Check sheet for the modelled part. Datum: model origin and axes. Units: mm. A direction names the side the tool comes from. Round coordinates to 2 decimals unless told otherwise and drop trailing zeros. Order: outer loops, then holes, each group sorted by start corner. A loop starts at its lowest first (then second) coordinate and runs counter-clockwise, first axis right, second up. Notation, with made-up numbers: M -11,-33.5 L 40,-33.5 A23 cw 40,-15.5 Z; hole C 60.25,19 d5. An arc over 180 degrees is marked long. One line per item, written item: value. Start each with the question number.
(1) Thickness scan on L1, parallel to Z at x = -73, y = 71; L2, parallel to X at y = 14, z = 7.75; L3, parallel to X at y = -11, z = 2.5. Record the ranges inside material, lowest first.
(2) Release check for a two-part mould opening along Z. For faces 3 (the face through (-80, 32, 8)), 4 (the face through (-78, -8.4, 12)) record: released by +Z, released by -Z, zero draft, split by the parting line, or undercut.
(3) Access from +Z, -Z, +X, -X, +Y, -Y to the whole of each face (thin tool, end or side, straight path). Record for faces 1 (the face through (-76.666, -33.778, -1.465)), 2 (the face through (-78, 53, 14)).
(4) Cross-section at A-A, the plane y = -32.5. Enter the section's corners in (x, z).
(5) Depth check by flat-ended pin: pin 1 Ø1.2 at (y, z) = (52, 2.5) entering from -X; pin 2 Ø2.5 at (x, y) = (-75, 52.5) entering from +Z. Enter the tip coordinate at first touch or a pass-through.
from build123d import *

# Parameters (mm, degrees)
SKETCH1_W           = 10
SKETCH1_H           = 85
BOSS_EXTRUDE2_DEPTH = 5
SKETCH2_W           = 10
SKETCH2_H           = 170
CUT_EXTRUDE1_DEPTH  = 1
SKETCH3_W           = 5
SKETCH3_H           = 8.2
CUT_EXTRUDE2_DEPTH  = 4
BOSS_EXTRUDE3_DEPTH = 9
SKETCH6_W           = 5
SKETCH6_H           = 170
BOSS_EXTRUDE4_DEPTH = 10
SKETCH7_W           = 10
SKETCH7_H           = 170
BOSS_EXTRUDE6_DEPTH = 5
SKETCH9_W           = 10
SKETCH9_H           = 170
BOSS_EXTRUDE7_DEPTH = 5
SKETCH10_R          = 2.1
CUT_EXTRUDE3_DEPTH  = 39
CUT_EXTRUDE6_DEPTH  = 39
SKETCH14_W          = 10
SKETCH14_H          = 2
CUT_EXTRUDE7_DEPTH  = 39


with BuildPart() as part:
    # Sketch1 → Boss-Extrude2 (new body)
    with BuildSketch(Plane.XY):
        with Locations((-75, 0)):
            Rectangle(SKETCH1_W, SKETCH1_H)
        Polygon((-78.6, 10.4), (-75, 8.4), (-71.4, 10.4), (-71.4, 14.6), (-75, 16.6), (-78.6, 14.6), align=None, mode=Mode.SUBTRACT)
        Polygon((-78.6, 34.6), (-78.6, 30.4), (-75, 28.4), (-71.4, 30.4), (-71.4, 34.6), (-75, 36.6), align=None, mode=Mode.SUBTRACT)
        Polygon((-78.6, -10.4), (-78.6, -14.6), (-75, -16.6), (-71.4, -14.6), (-71.4, -10.4), (-75, -8.4), align=None, mode=Mode.SUBTRACT)
        Polygon((-78.6, -34.6), (-75, -36.6), (-71.4, -34.6), (-71.4, -30.4), (-75, -28.4), (-78.6, -30.4), align=None, mode=Mode.SUBTRACT)
        with Locations((-75, 85)):
            Rectangle(SKETCH1_W, SKETCH1_H)
        Polygon((-78.6, 115.4), (-75, 113.4), (-71.4, 115.4), (-71.4, 119.6), (-75, 121.6), (-78.6, 119.6), align=None, mode=Mode.SUBTRACT)
        Polygon((-78.6, 95.4), (-75, 93.4), (-71.4, 95.4), (-71.4, 99.6), (-75, 101.6), (-78.6, 99.6), align=None, mode=Mode.SUBTRACT)
        Polygon((-78.6, 50.4), (-75, 48.4), (-71.4, 50.4), (-71.4, 54.6), (-75, 56.6), (-78.6, 54.6), align=None, mode=Mode.SUBTRACT)
        Polygon((-78.6, 74.6), (-78.6, 70.4), (-75, 68.4), (-71.4, 70.4), (-71.4, 74.6), (-75, 76.6), align=None, mode=Mode.SUBTRACT)
    extrude(amount=BOSS_EXTRUDE2_DEPTH)

    # Sketch2 → Cut-Extrude1 (cut)
    with BuildSketch(Plane(origin=(0, 0, 0), x_dir=(-1, 0, 0), z_dir=(0, 0, -1))):
        with Locations((75, 42.5)):
            Rectangle(SKETCH2_W, SKETCH2_H)
    extrude(amount=-CUT_EXTRUDE1_DEPTH, mode=Mode.SUBTRACT)

    # Sketch3 → Cut-Extrude2 (cut)
    with BuildSketch(Plane(origin=(0, 0, 1), x_dir=(-1, 0, 0), z_dir=(0, 0, -1))):
        with Locations((77.5, 117.5)):
            Rectangle(SKETCH3_W, SKETCH3_H)
        with Locations((77.5, 97.5)):
            Rectangle(SKETCH3_W, SKETCH3_H)
        with Locations((77.5, 72.5)):
            Rectangle(SKETCH3_W, SKETCH3_H)
        with Locations((77.5, 52.5)):
            Rectangle(SKETCH3_W, SKETCH3_H)
        with Locations((77.5, 32.5)):
            Rectangle(SKETCH3_W, SKETCH3_H)
        with Locations((77.5, 12.5)):
            Rectangle(SKETCH3_W, SKETCH3_H)
        with Locations((77.5, -12.5)):
            Rectangle(SKETCH3_W, SKETCH3_H)
        with Locations((77.5, -32.5)):
            Rectangle(SKETCH3_W, SKETCH3_H)
    extrude(amount=-CUT_EXTRUDE2_DEPTH, mode=Mode.SUBTRACT)

    # Sketch5 → Boss-Extrude3 (add)
    with BuildSketch(Plane.XY.offset(5)):
        Polygon((-70, 127.5), (-80, 127.5), (-80, 121.6), (-75, 121.6), (-71.4, 119.6), (-71.4, 115.4), (-75, 113.4), (-80, 113.4), (-80, 101.6), (-75, 101.6), (-71.4, 99.6), (-71.4, 95.4), (-75, 93.4), (-80, 93.4), (-80, 76.6), (-75, 76.6), (-71.4, 74.6), (-71.4, 70.4), (-75, 68.4), (-80, 68.4), (-80, 56.6), (-75, 56.6), (-71.4, 54.6), (-71.4, 50.4), (-75, 48.4), (-80, 48.4), (-80, 36.6), (-75, 36.6), (-71.4, 34.6), (-71.4, 30.4), (-75, 28.4), (-80, 28.4), (-80, 16.6), (-75, 16.6), (-71.4, 14.6), (-71.4, 10.4), (-75, 8.4), (-80, 8.4), (-80, -8.4), (-75, -8.4), (-71.4, -10.4), (-71.4, -14.6), (-75, -16.6), (-80, -16.6), (-80, -28.4), (-75, -28.4), (-71.4, -30.4), (-71.4, -34.6), (-75, -36.6), (-80, -36.6), (-80, -42.5), (-70, -42.5), align=None)
    extrude(amount=BOSS_EXTRUDE3_DEPTH)

    # Sketch6 → Boss-Extrude4 (add)
    with BuildSketch(Plane.ZY.offset(80)):
        with Locations((7.5, 42.5)):
            Rectangle(SKETCH6_W, SKETCH6_H)
    extrude(amount=-BOSS_EXTRUDE4_DEPTH)

    # Sketch7 → Boss-Extrude6 (add)
    with BuildSketch(Plane.XY.offset(14)):
        with Locations((-75, 42.5)):
            Rectangle(SKETCH7_W, SKETCH7_H)
    extrude(amount=BOSS_EXTRUDE6_DEPTH)

    # Sketch9 → Boss-Extrude7 (add)
    with BuildSketch(Plane(origin=(0, 0, 1), x_dir=(-1, 0, 0), z_dir=(0, 0, -1))):
        with Locations((75, 42.5)):
            Rectangle(SKETCH9_W, SKETCH9_H)
    extrude(amount=BOSS_EXTRUDE7_DEPTH)

    # Sketch10 → Cut-Extrude3 (cut)
    with BuildSketch(Plane.XY.offset(19)):
        with Locations((-75, 117.5)):
            Circle(SKETCH10_R)
        with Locations((-75, 97.5)):
            Circle(SKETCH10_R)
        with Locations((-75, 72.5)):
            Circle(SKETCH10_R)
        with Locations((-75, 52.5)):
            Circle(SKETCH10_R)
        with Locations((-75, 32.5)):
            Circle(SKETCH10_R)
        with Locations((-75, 12.5)):
            Circle(SKETCH10_R)
        with Locations((-75, -12.5)):
            Circle(SKETCH10_R)
        with Locations((-75, -32.5)):
            Circle(SKETCH10_R)
    extrude(amount=-CUT_EXTRUDE3_DEPTH, mode=Mode.SUBTRACT)

    # Sketch13 → Cut-Extrude6 (cut)
    with BuildSketch(Plane(origin=(0, 0, -4), x_dir=(-1, 0, 0), z_dir=(0, 0, -1))):
        Polygon((70, 127.5), (75, 127.5), (80, 127.5), (80, 107.5), (75, 107.5), (70, 107.5), align=None)
    extrude(amount=-CUT_EXTRUDE6_DEPTH, mode=Mode.SUBTRACT)

    # Sketch14 → Cut-Extrude7 (cut)
    with BuildSketch(Plane(origin=(0, 0, -4), x_dir=(-1, 0, 0), z_dir=(0, 0, -1))):
        with Locations((75, -41.5)):
            Rectangle(SKETCH14_W, SKETCH14_H)
    extrude(amount=-CUT_EXTRUDE7_DEPTH, mode=Mode.SUBTRACT)


solid = part.part
Values found:
1. L1: -4 to 1, 5 to 10, 14 to 19
1. L2: -80 to -76.47, -73.53 to -70
1. L3: -71.4 to -70
2. face 3: zero draft
2. face 4: undercut
3. face 1: +Z, -Z
3. face 2: -X
4. outline: M -80,-4 L -77.1,-4 L -77.1,1 L -80,1 Z; M -80,5 L -77.1,5 L -77.1,10 L -80,10 Z; M -80,14 L -77.1,14 L -77.1,19 L -80,19 Z; M -72.9,-4 L -70,-4 L -70,19 L -72.9,19 L -72.9,14 L -71.4,14 L -71.4,10 L -72.9,10 L -72.9,5 L -71.4,5 L -71.4,1 L -72.9,1 Z
5. pin 1: x = -71.4
5. pin 2: through
